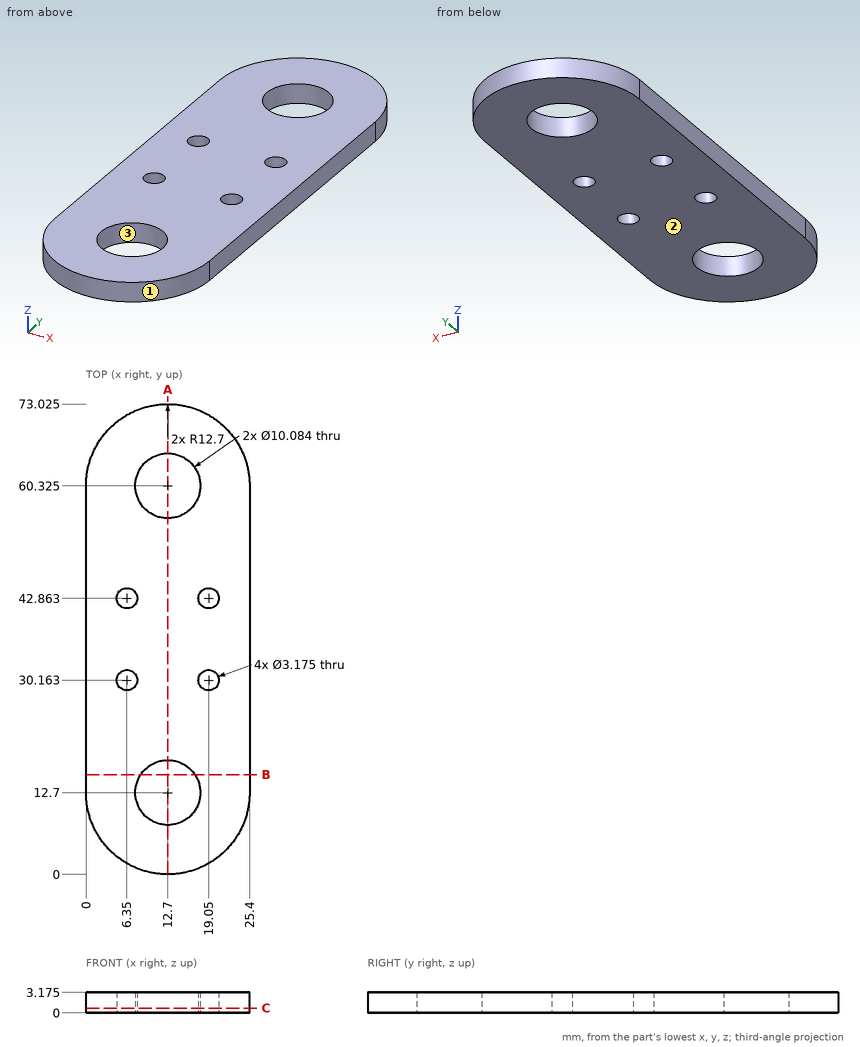
Study the drawing (mm; zero at the part's minimum x, y, z) and answer. Round coordinates to 2 decimals unless told otherwise and drop trailing zeros. Write each loop counter-clockwise with the first axis right and the second up, starting at its lowest first coordinate (ties: lowest second). Pieces come first, ordered by that corner, then holes.
1) A cutting plane is placed at C-C on z = 0.75. Give the number of separate pieces and of enclosed holes in the cut face, and give its area (4 significant figures).
2) A cutting plane is placed at A-A on x = 12.7. Determine the outline of the cut face in (y, z) (1 decimal), and give its area (3 significant figures).
3) Determine the mould class of the marked faces 1, 2 and 3 for opening direction X: pulls with the +X half, pulls with the -X half, needs draft (parallel to the pull), parting line crosses it, or undercut.
4) A cutting plane is placed at B-B on y = 15.5. Determine the outline of the cut face in (x, z) (1 decimal).
5) Consider probe 1 along Y at (x, z) = (12.7, 2.45) (1 decimal); probe 2 along X at (y, z) = (43, 1.8); probe 3 along Y at (x, z) = (5.25, 3) (1 decimal). Determine where each line is inside the solid, lowest interval first.
Entries:
1. separate pieces: 1
1. enclosed holes: 6
1. area: 1,525 mm2
2. outline: (0, 0) - (7.7, 0) - (7.7, 3.2) - (0, 3.2) - close; (17.7, 0) - (55.3, 0) - (55.3, 3.2) - (17.7, 3.2) - close; (65.4, 0) - (73, 0) - (73, 3.2) - (65.4, 3.2) - close
2. area: 168 mm2
3. face 1: parting line crosses it
3. face 2: needs draft
3. face 3: undercut
4. outline: (0, 0) - (8.5, 0) - (8.5, 3.2) - (0, 3.2) - close; (16.9, 0) - (25.4, 0) - (25.4, 3.2) - (16.9, 3.2) - close
5. probe 1: y = 0 to 7.7, 17.7 to 55.3, 65.4 to 73
5. probe 2: x = 0 to 4.77, 7.93 to 17.47, 20.63 to 25.4
5. probe 3: y = 2.4 to 29, 31.3 to 41.7, 44 to 70.6
